from build123d import *

# Parameters (mm, degrees)
F0_R     = 497.5
F0_R_2   = 416.5
F1_DEPTH = 32
F2_R     = 445
F2_R_2   = 425
F3_DEPTH = 123
F6_R     = 9
F7_DEPTH = 155.001


with BuildPart() as f1:
    # F0 (on Top) → F1 (new body)
    with BuildSketch(Plane.XY):
        Circle(F0_R)
        Circle(F0_R_2, mode=Mode.SUBTRACT)
    extrude(amount=F1_DEPTH)

    # F2 (on face) → F3 (join)
    with BuildSketch(Plane.XY.offset(32)):
        Circle(F2_R)
        Circle(F2_R_2, mode=Mode.SUBTRACT)
    extrude(amount=F3_DEPTH)

    # F4 (on Right) → F5 (revolve, cut)
    with BuildSketch(Plane.YZ):
        Polygon((-445, 155), (-445, 145.5), (-435.5, 155), align=None)
        Polygon((-425, 155), (-434.5, 155), (-425, 145.5), align=None)
    revolve(axis=Axis((0, 0, 155), (0, 0, 1)), mode=Mode.SUBTRACT)

    # F6 (on face) → F7 (cut, through all)
    with BuildSketch(Plane(origin=(0, 0, 0), x_dir=(1, 0, 0), z_dir=(0, 0, -1))):
        with Locations((0, 469)):
            Circle(F6_R)
        with Locations((73.367764, 463.225832)):
            Circle(F6_R)
        with Locations((144.92897, 446.045506)):
            Circle(F6_R)
        with Locations((212.921544, 417.88206)):
            Circle(F6_R)
        with Locations((275.671283, 379.42897)):
            Circle(F6_R)
        with Locations((331.63308, 331.63308)):
            Circle(F6_R)
        with Locations((379.42897, 275.671283)):
            Circle(F6_R)
        with Locations((417.88206, 212.921544)):
            Circle(F6_R)
        with Locations((446.045506, 144.92897)):
            Circle(F6_R)
        with Locations((463.225832, 73.367764)):
            Circle(F6_R)
        with Locations((469, 0)):
            Circle(F6_R)
        with Locations((463.225832, -73.367764)):
            Circle(F6_R)
        with Locations((446.045506, -144.92897)):
            Circle(F6_R)
        with Locations((417.88206, -212.921544)):
            Circle(F6_R)
        with Locations((379.42897, -275.671283)):
            Circle(F6_R)
        with Locations((331.63308, -331.63308)):
            Circle(F6_R)
        with Locations((275.671283, -379.42897)):
            Circle(F6_R)
        with Locations((212.921544, -417.88206)):
            Circle(F6_R)
        with Locations((144.92897, -446.045506)):
            Circle(F6_R)
        with Locations((73.367764, -463.225832)):
            Circle(F6_R)
        with Locations((0, -469)):
            Circle(F6_R)
        with Locations((-73.367764, -463.225832)):
            Circle(F6_R)
        with Locations((-144.92897, -446.045506)):
            Circle(F6_R)
        with Locations((-212.921544, -417.88206)):
            Circle(F6_R)
        with Locations((-275.671283, -379.42897)):
            Circle(F6_R)
        with Locations((-331.63308, -331.63308)):
            Circle(F6_R)
        with Locations((-379.42897, -275.671283)):
            Circle(F6_R)
        with Locations((-417.88206, -212.921544)):
            Circle(F6_R)
        with Locations((-463.225832, -73.367764)):
            Circle(F6_R)
        with Locations((-469, 0)):
            Circle(F6_R)
        with Locations((-463.225832, 73.367764)):
            Circle(F6_R)
        with Locations((-446.045506, 144.92897)):
            Circle(F6_R)
        with Locations((-417.88206, 212.921544)):
            Circle(F6_R)
        with Locations((-379.42897, 275.671283)):
            Circle(F6_R)
        with Locations((-331.63308, 331.63308)):
            Circle(F6_R)
        with Locations((-275.671283, 379.42897)):
            Circle(F6_R)
        with Locations((-212.921544, 417.88206)):
            Circle(F6_R)
        with Locations((-144.92897, 446.045506)):
            Circle(F6_R)
        with Locations((-73.367764, 463.225832)):
            Circle(F6_R)
    extrude(amount=-F7_DEPTH, mode=Mode.SUBTRACT)


solid = f1.part
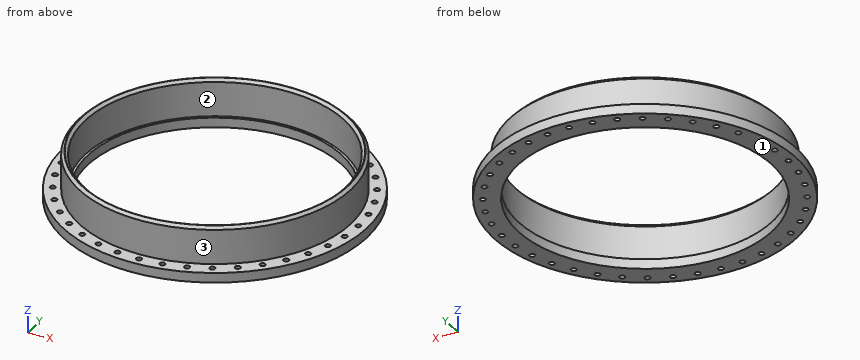
Source: CAD feature listing. Evaluate the final solid. Frame: model axes, mm. Face numbers are marked on the shaded views. Coordinates: 2 decimals unless noted, no trailing zeros. Loops run counter-clockwise (first coordinate to the right, second up) from the corner with the lowest first, then second, coordinate; pieces in that order, holes last. Notation, with made-up numbers: (67.5, 28) -> (114.5, 28) arc R29 ccw to (114.5, 66) -> close; hole circle Ø7 at (45.25, 79). An arc over 180 degrees is marked (long way). Answer in a Markdown table with one row per item. Add a question column.
Q1. Ray query, line 1 along X through (y, z) = (261.5, 46); line 2 along Y through (x, z) = (-161.5, 147); line 3 along Y through (x, z) = (279, 92). Return the intervals inside material, ascending.
Q2. Section B-B on z = 15.5. Give the number of separate pieces and of enclosed holes in the cut face, and give its area (3 significant figures).
Q3. Contact query for flat-ended pins moving along their axis: pin 1 Ø12 at (y, z) = (232.5, 63.5) entering from -X; pin 2 Ø2 at (x, z) = (-331, 62.5) entering from +Y; pin 3 Ø1 at (x, z) = (342.5, 107.5) entering from +Y. Output: stop coordinate, or through.
Q4. Section A-A on z = 84. Return the cut outline in (x, y), and give its area (3 significant figures).
Q5. Pull-direction query (X, two-part tool) for the marked faces 1, 2 and 3; classes: pulls with the +X half, pulls with the -X half, needs draft (parallel to the pull), parting line crosses it, or undercut.
Computed values:
| question | item | result |
|---|---|---|
| 1 | line 1 | x = -360.06 to -335.03, 335.03 to 360.06 |
| 1 | line 2 | y = -413.05 to -394.74, 394.74 to 413.05 |
| 1 | line 3 | y = -346.68 to -320.6, 320.6 to 346.68 |
| 2 | separate pieces | 1 |
| 2 | enclosed holes | 40 |
| 2 | area | 223,000 mm^2 |
| 3 | pin 1 | stops at x = -383.04 |
| 3 | pin 2 | stops at y = 298.54 |
| 3 | pin 3 | stops at y = 284.71 |
| 4 | outline | circle Ø890 at (0, 0); hole circle Ø850 at (0, 0) |
| 4 | area | 54,700 mm^2 |
| 5 | face 1 | needs draft |
| 5 | face 2 | undercut |
| 5 | face 3 | parting line crosses it |
